Autodesk Inventor part; units mm, degrees
ref_plane "YZ Plane" through (0, 0, 0) normal (1, 0, 0) x (0, 1, 0)
ref_plane "XZ Plane" through (0, 0, 0) normal (0, 1, 0) x (-1, 0, 0)
ref_plane "XY Plane" through (0, 0, 0) normal (0, 0, 1) x (1, 0, 0)
sketch "Esquisse2" plane through (0, 0, 0) normal (0, 1, 0) x (-1, 0, 0)
  line L0 (10, -10) -> (-10, -10)
  line L1 (-10, -10) -> (-10, 10)
  line L2 (-10, 10) -> (10, 10)
  line L3 (10, 10) -> (10, -10)
  line L4 (10, -10) -> (-10, 10) construction
  line L5 (-10, -10) -> (10, 10) construction
  point P0 (0, 0)
  dimension "d6" = 20
  dimension "d7" = 20
extrude "Extrusion1" add sketch "Esquisse2" along normal blind 40
sketch "Esquisse3" plane through (0, 0, 0) normal (0, 0, 1) x (1, 0, 0)
  line L0 (-10, 40) -> (10, 40)
  line L1 (15, 88) -> (15, 42)
  line L2 (13, 40) -> (-13, 40)
  line L3 (-15, 42) -> (-15, 88)
  line L4 (-15, 90) -> (15, 40) construction
  line L5 (15, 90) -> (-15, 40) construction
  line L6 (13, 90) -> (4.8464, 90)
  line L7 (-4.8464, 90) -> (-13, 90)
  line L8 (-15, 90) -> (-3, 90)
  line L9 (3, 90) -> (15, 90)
  line L10 (-2.8528, 88.1595) -> (-2.1472, 79.3405)
  line L11 (-0.1536, 77.5) -> (0.1536, 77.5)
  line L12 (2.1472, 79.3405) -> (2.8528, 88.1595)
  arc A0 (-13, 90) -> (-15, 88) centre (-13, 88) ccw
  arc A1 (15, 88) -> (13, 90) centre (13, 88) ccw
  arc A2 (-2.1472, 79.3405) -> (-0.1536, 77.5) centre (-0.1536, 79.5) ccw
  arc A3 (0.1536, 77.5) -> (2.1472, 79.3405) centre (0.1536, 79.5) ccw
  arc A4 (-2.8528, 88.1595) -> (-4.8464, 90) centre (-4.8464, 88) ccw
  arc A5 (4.8464, 90) -> (2.8528, 88.1595) centre (4.8464, 88) ccw
  arc A6 (-15, 42) -> (-13, 40) centre (-13, 42) ccw
  arc A7 (13, 40) -> (15, 42) centre (13, 42) ccw
  point P0 (0, 0)
  point P1 (0, 65)
  point P2 (-2, 77.5)
  point P3 (2, 77.5)
  dimension "d10" = 30
  dimension "d11" = 50
  dimension "d12" = 0
  dimension "d23" = 12
  dimension "d24" = 12
  dimension "d27" = 4
  dimension "d28" = 1
  dimension "d29" = 37.5
  dimension "d30" = 2
extrude "Extrusion2" add sketch "Esquisse3" along normal mid plane 35
sketch "Esquisse5" plane through (15, 42, 17.5) normal (1, 0, 0) x (0, 0, -1)
  line L0 (5, 61.6074) -> (30, 61.6074)
  line L1 (30, 61.6074) -> (30, 6)
  line L2 (27, 3) -> (8, 3)
  line L3 (5, 6) -> (5, 61.6074)
  line L4 (5, 61.6074) -> (30, 3) construction
  line L5 (30, 61.6074) -> (5, 3) construction
  line L6 (35, 46) -> (35, 0)
  line L7 (35, -2) -> (0, -2)
  line L8 (0, 0) -> (0, 46)
  arc A0 (5, 6) -> (8, 3) centre (8, 6) ccw
  arc A1 (27, 3) -> (30, 6) centre (27, 6) ccw
  point P0 (17.5, -42)
  point P1 (17.5, 32.3037)
  dimension "d31" = 5
  dimension "d32" = 5
  dimension "d33" = 5
  dimension "d34" = 3
extrude "Extrusion4" cut sketch "Esquisse5" against normal blind 35
sketch "Esquisse6" plane through (0, 0, 0) normal (0, 0, 1) x (1, 0, 0)
  circle A0 centre (0, 80) radius 27.5
  line L0 (13, 40) -> (-13, 40)
  point P0 (0, 0)
  dimension "d37" = 55
  dimension "d38" = 40
extrude "Extrusion5" add sketch "Esquisse6" along normal mid plane 20
sketch "Esquisse7" plane through (0, 80, -10) normal (0, 0, -1) x (-1, 0, 0)
  circle A0 centre (0, -0.6595) radius 2.1404
  line L0 (-2.1472, -0.6595) -> (-2.8528, 8.1595)
  point P0 (0, -80)
extrude "Extrusion6" add sketch "Esquisse7" along normal blind 10 and the other way blind 30
properties part number "RouleauTendeur"
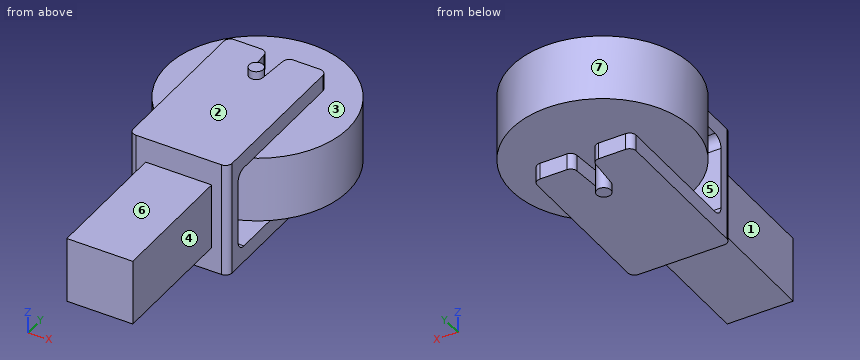
Work out the finished part from the listing and answer in its coordinate system (mm). Face numbers are marked on the shaded views. A direction names the side the tool comes from. Coordinates: 2 decimals unless noted, no trailing zeros. Loops run counter-clockwise (first coordinate to the right, second up) from the corner with the lowest first, then second, coordinate; pieces in that order, holes last.
1) Section B-B (x = -8) is taken. Give the vertices of the cut face in (y, z), plus the area to 3 significant figures.
Results:
outline: (0, -10) - (40, -10) - (40, -17.5) - (90, -17.5) - (90, -12.5) - (48, -12.5) arc R3 cw to (45, -9.5) - (45, 9.5) arc R3 cw to (48, 12.5) - (90, 12.5) - (90, 17.5) - (40, 17.5) - (40, 10) - (0, 10) - close; (53.69, -10) - (106.31, -10) - (106.31, 10) - (53.69, 10) - close
area: 2,480 mm2
2) Section C-C (y = 66) is taken. Give the vertices of the cut face in (x, z), plus the area to 3 significant figures.
Results:
outline: (-23.67, -10) - (23.67, -10) - (23.67, 10) - (-23.67, 10) - close; (-15, -17.5) - (15, -17.5) - (15, -12.5) - (-15, -12.5) - close; (-15, 12.5) - (15, 12.5) - (15, 17.5) - (-15, 17.5) - close
area: 1,250 mm2
3) For the marked faces 4, 5, 6 and 7, determine the directions among +Z, -Z, +X, -X, +Y, -Y from which every point of the face is accessible in a straight line to the end or side of a thin tool.
Results:
face 4: +Z, -Z, +X, -Y
face 5: +X, -X
face 6: +Z, +X, -X, -Y
face 7: none
4) Consider probe 1 along Z at (x, y) = (10, 75); probe 2 along X at (y, z) = (47, 13.5); probe 3 along Z at (x, y) = (22, 78). Determine where each line is inside the solid, lowest interval first.
Results:
probe 1: z = -17.5 to -12.5, -10 to 10, 12.5 to 17.5
probe 2: x = -15 to 15
probe 3: z = -10 to 10
5) Section A-A (z = -4.5) is taken. Give the vertices of the cut face in (x, y).
Results:
outline: circle Ø55 at (0, 80); (-15, 42) arc R2 ccw to (-13, 40) - (-10, 40) - (-10, 0) - (10, 0) - (10, 40) - (13, 40) arc R2 ccw to (15, 42) - (15, 45) - (-15, 45) - close
6) Flat-ended cylindrical pins translate along their axes: pin 1 (2 mm diameter, centred on x = -6.5, z = -7, fed in from -Y); pin 2 (2 mm diameter, centred on y = 23, z = 10, fed in from +X); pin 3 (15 mm diameter, centred on x = 1, y = 68.5, fed in from -Z); pin 4 (2.5 mm diameter, centred on x = -9.5, z = 15.5, fed in from +Y). Find the tip coordinate at first contact, or state that the pin passes through.
Results:
pin 1: stops at y = 0
pin 2: stops at x = 10
pin 3: stops at z = -17.5
pin 4: stops at y = 90
7) For a pull along Z with two mould halves and no side action, classify the marked faces 1, 2 and 3 as +Z half, -Z half, draft (parallel to the pull), parting line (faces both ways), or undercut.
Results:
face 1: draft
face 2: +Z half
face 3: undercut
8) Section D-D (z = -14.5) is taken. Give the vertices of the cut face in (x, y).
Results:
outline: (-15, 42) arc R2 ccw to (-13, 40) - (13, 40) arc R2 ccw to (15, 42) - (15, 88) arc R2 ccw to (13, 90) - (4.85, 90) arc R2 ccw to (2.85, 88.16) - (2.15, 79.34) arc R2 cw to (2.14, 79.26) arc R2.14 ccw (long way) to (-2.14, 79.26) arc R2 cw to (-2.15, 79.34) - (-2.85, 88.16) arc R2 ccw to (-4.85, 90) - (-13, 90) arc R2 ccw to (-15, 88) - close
